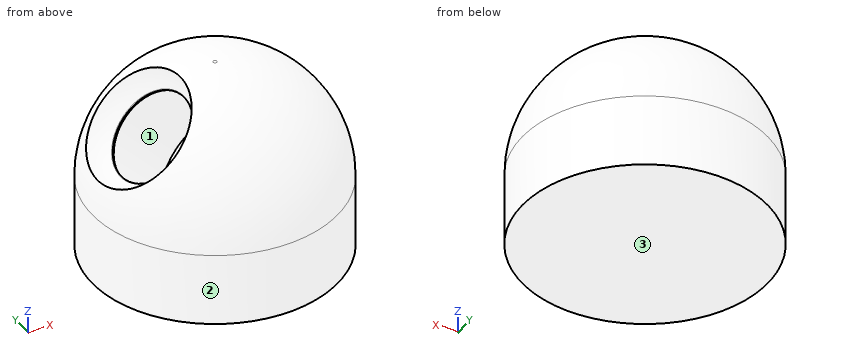
from build123d import *

# Parameters (mm, degrees)
F0_R     = 12.7
F1_DEPTH = 20
F2_R     = 12.5


# Not quite as in the source:
# - a fillet or chamfer that OpenCascade refuses, or shapes differently, is made with other operations: its cross-section is extruded or revolved along the edge and cut away or added


with BuildPart() as f1:
    # F0 (on Top) → F1 (new body)
    with BuildSketch(Plane.XY):
        Circle(F0_R)
    extrude(amount=F1_DEPTH)

    # F2
    f2_edges = [f1.edges().sort_by_distance(p)[0] for p in [
        (-12.7, 0, 20),
    ]]
    fillet(f2_edges, radius=F2_R)

    # F3 (on Front) → F4 (revolve, cut)
    with BuildSketch(Plane.XZ):
        Polygon((6.0710678119, 11.9289321881), (-1, 19), (-6.25, 13.75), (0.8210678119, 6.6789321881), align=None)
    revolve(axis=Axis((-2.7144660941, 0, 10.2144660941), (0.7071067812, 0, -0.7071067812)), mode=Mode.SUBTRACT)

    # F5 (on Front) → F6 (revolve, cut)
    with BuildSketch(Plane.XZ):
        with BuildLine():
            Line((-9.7855339059, 17.2855339059), (-5.1186291501, 12.6186291501))
            ThreePointArc((-5.1186291501, 12.6186291501), (-3.6879289914, 14.7598232523), (-3.1855339059, 17.2855339059))
            ThreePointArc((-3.1855339059, 17.2855339059), (-7.2598232523, 23.3831388205), (-14.4524386618, 21.9524386618))
            Line((-14.4524386618, 21.9524386618), (-9.7855339059, 17.2855339059))
        make_face()
    revolve(axis=Axis((-12.1189862838, 0, 19.6189862838), (-0.7071067812, 0, 0.7071067812)), mode=Mode.SUBTRACT)

    # F7: chamfer of 0.4 on 1 edges, made by hand

    # F7_s1 → F7_t2 (revolve, cut)
    with BuildSketch(Plane.XZ):
        with BuildLine():
            Line((-3.2011954465, 17.1809028584), (-2.9181547597, 17.0608682325))
            Line((-2.9181547597, 17.0608682325), (-2.9124979054, 17.0552113782))
            ThreePointArc((-2.9124979054, 17.0552113782), (-3.0605101564, 16.9281761351), (-3.1980339034, 16.7906523881))
            Line((-3.1980339034, 16.7906523881), (-3.2116687493, 16.7969022419))
            ThreePointArc((-3.2116687493, 16.7969022419), (-3.2002291645, 16.9885061916), (-3.2091943175, 17.1810372559))
            Line((-3.2091943175, 17.1810372559), (-3.2011954465, 17.1809028584))
        make_face()
    revolve(axis=Axis((-6.25, 0, 13.75), (-0.7071067812, 0, 0.7071067812)), mode=Mode.SUBTRACT)


solid = f1.part
Geometry: final body of the model. Coordinates: model frame, mm. Face numbers are marked on the shaded views. Give positions to 0.01 mm unless a question says otherwise; leave off trailing zeros. Answer as a JSON object with one key per item and string values.
Q1. Draft query along Z for the marked faces 1, 2 and 3. Return one class per face: released by +Z, released by -Z, zero draft, split by the parting line, or undercut.
Entries:
{"face 1": "undercut", "face 2": "zero draft", "face 3": "released by -Z"}
Q2. First-contact query: pin 1 (8 mm diameter, centred on x = -8, y = -6, fed in from -Z); pin 2 (2 mm diameter, centred on y = -2.5, z = 5, fed in from +X); pin 3 (4 mm diameter, centred on x = -9, y = 4, fed in from +Z); pin 4 (6 mm diameter, centred on y = 2.5, z = 16.5, fed in from +X). Flat tips, straight axial feed; report the tip coordinate or a pass-through.
Entries:
{"pin 1": "stops at z = 0", "pin 2": "stops at x = 12.61", "pin 3": "stops at z = 14.71", "pin 4": "stops at x = 10.97"}
Q3. Material intervals for probe 1 along Y at (x, z) = (-3, 11.5); probe 2 along Y at (x, z) = (2.25, 15.25); probe 3 along Z at (x, y) = (3.75, 2), sorted ascending.
Entries:
{"probe 1": "y = -11.66 to -7.39, 7.39 to 11.66", "probe 2": "y = -9.75 to -2.26, 2.26 to 9.75", "probe 3": "z = 0 to 9.61, 13.86 to 19.33"}
